from build123d import *

# Parameters (mm, degrees)
SKETCH1_R           = 1.5621
SKETCH1_W           = 6.35
SKETCH1_H           = 12.7
BOSS_EXTRUDE1_DEPTH = 6.35


with BuildPart() as part:
    # Sketch1 → Boss-Extrude1 (new body)
    with BuildSketch(Plane(origin=(0, 0, 0), x_dir=(1, 0, 0), z_dir=(0, 1, 0))):
        Polygon((-29.684698321, 16.343647987), (29.684698321, 16.343647987), (31.0388, 16.343647987), (31.0388, -16.343647987), (29.684698321, -16.343647987), (-29.684698321, -16.343647987), (-31.0388, -16.343647987), (-31.0388, 16.343647987), align=None)
        with Locations((-24.709647151, 11.044056729)):
            Circle(SKETCH1_R, mode=Mode.SUBTRACT)
        with Locations((-24.709647151, -11.044056729)):
            Circle(SKETCH1_R, mode=Mode.SUBTRACT)
        with Locations((24.709647151, 11.044056729)):
            Circle(SKETCH1_R, mode=Mode.SUBTRACT)
        with Locations((24.709647151, -11.044056729)):
            Circle(SKETCH1_R, mode=Mode.SUBTRACT)
        with Locations((24.6888, -0.068443271)):
            Rectangle(SKETCH1_W, SKETCH1_H, mode=Mode.SUBTRACT)
        with Locations((-24.6888, -0.068443271)):
            Rectangle(SKETCH1_W, SKETCH1_H, mode=Mode.SUBTRACT)
    extrude(amount=BOSS_EXTRUDE1_DEPTH)


solid = part.part
Here's how the part is built. I have some questions about the finished solid (model axes, mm). A direction names the side the tool comes from. Give positions to 0.01 mm unless a question says otherwise; leave off trailing zeros. Write each loop counter-clockwise with the first axis right and the second up, starting at its lowest first coordinate (ties: lowest second). Pieces come first, ordered by that corner, then holes. Notation, with made-up numbers: (65.5, 87.5) -> (99.5, 87.5) arc R16 cw to (99.5, 109.5) -> close; hole circle Ø9 at (25.5, 75). An arc over 180 degrees is marked (long way). Use one line per item in the form item = value. Start each with the question number.
1. Imagine slicing it at C-C on y = 3.25. List the corners of the cut face in (x, z) for me, plus the area to 3 significant figures.
2. On a 3-axis mill with a long thin cutter (end or side, diameter ignored), from which of +Z, -Z, +X, -X, +Y, -Y can I reach the whole of each face in a straight line? I mean faces 1 (the face through (-25, 3, 6.418)), 2 (the face through (0, 0, 0)). Say none if no direction works.
3. If I drill on L1, parallel to X at y = 1.5, z = 2.5; L2, parallel to X at y = 3.25, z = 10; L3, parallel to Z at x = -23.5, y = 5.75, over which ranges is the centre line in solid material (lowest first)?
4. Will this pin go through, and if not, where does the flat tip stop? pin 1 Ø2.5 at (x, z) = (-24.71, -11.04) entering from +Y.
5. Imagine slicing it at B-B on z = 12. List the corners of the cut face in (x, y) for me.
6. Imagine slicing it at A-A on x = -24.5. List the corners of the cut face in (y, z) for me, plus the area to 3 significant figures.
7. Thinking about a two-plate mould opening in Z: for faces 3 (the face through (27.864, 3, 0)), 4 (the face through (0, 3, 16.344)), 5 (the face through (31.039, 3, 0)), 6 (the face through (0, 3, -16.344)), which applies, +Z half, -Z half, draft (parallel to the pull), parting line (faces both ways), or undercut?
Entries:
q1.outline = (-31.04, -16.34) -> (31.04, -16.34) -> (31.04, 16.34) -> (-31.04, 16.34) -> close; hole (-27.86, -6.28) -> (-21.51, -6.28) -> (-21.51, 6.42) -> (-27.86, 6.42) -> close; hole circle Ø3.12 at (-24.71, -11.04); hole circle Ø3.12 at (-24.71, 11.04); hole (21.51, -6.28) -> (27.86, -6.28) -> (27.86, 6.42) -> (21.51, 6.42) -> close; hole circle Ø3.12 at (24.71, -11.04); hole circle Ø3.12 at (24.71, 11.04)
q1.area = 1,840 mm²
q2.face_1 = +Y, -Y
q2.face_2 = +Z, -Z, +X, -X, -Y
q3.L1 = -31.04 to -27.86, -21.51 to 21.51, 27.86 to 31.04
q3.L2 = -31.04 to -25.87, -23.55 to 23.55, 25.87 to 31.04
q3.L3 = -16.34 to -12.03, -10.06 to -6.28, 6.42 to 10.06, 12.03 to 16.34
q4.pin_1 = through
q5.outline = (-31.04, 0) -> (-25.95, 0) -> (-25.95, 6.35) -> (-31.04, 6.35) -> close; (-23.47, 0) -> (23.47, 0) -> (23.47, 6.35) -> (-23.47, 6.35) -> close; (25.95, 0) -> (31.04, 0) -> (31.04, 6.35) -> (25.95, 6.35) -> close
q6.outline = (0, -16.34) -> (6.35, -16.34) -> (6.35, -12.59) -> (0, -12.59) -> close; (0, -9.5) -> (6.35, -9.5) -> (6.35, -6.28) -> (0, -6.28) -> close; (0, 6.42) -> (6.35, 6.42) -> (6.35, 9.5) -> (0, 9.5) -> close; (0, 12.59) -> (6.35, 12.59) -> (6.35, 16.34) -> (0, 16.34) -> close
q6.area = 87.6 mm²
q7.face_3 = undercut
q7.face_4 = +Z half
q7.face_5 = draft
q7.face_6 = -Z half
